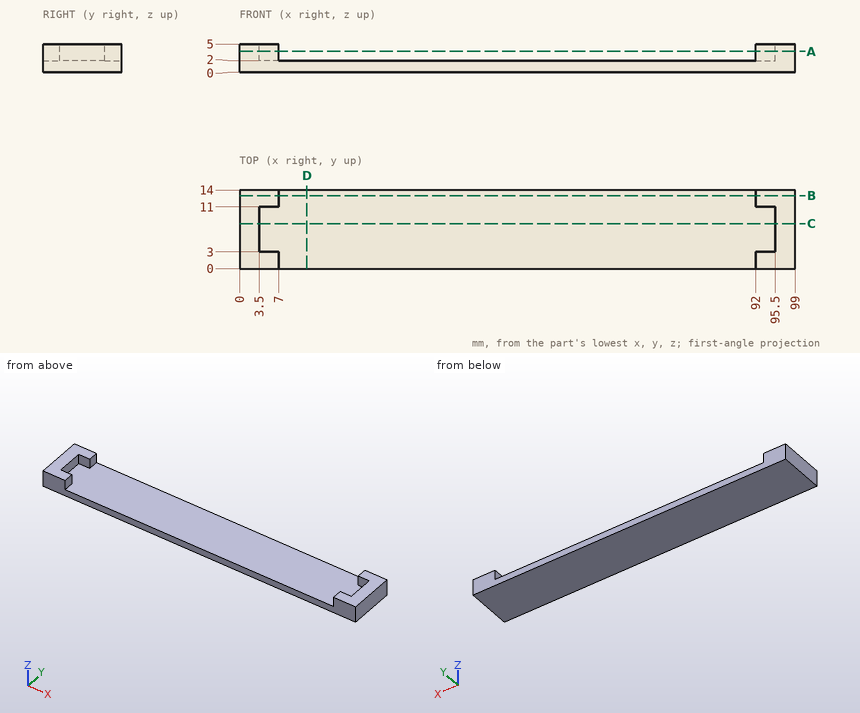
Geometry: see drawing. Coordinates: mm, zero at the bounding-box minimum. Round coordinates to 2 decimals unless told otherwise and drop trailing zeros. Loops run counter-clockwise (first coordinate to the right, second up) from the corner with the lowest first, then second, coordinate; pieces in that order, holes last. Notation, with made-up numbers: M -26,88 L -1,88 A32 cw -1,118 Z; hole C 62,12 d9. An arc over 180 degrees is marked long. Use a Markdown table: item, result. Add a question column.
1. Line query: line 1 (X direction, y = 6.5, z = 4.7); line 2 (X direction, y = 13.75, z = 4.05); line 3 (Z direction, x = 86.5, y = 8.75). Output: solid intervals per line, ascending.
2. Section query C-C on y = 8. Return the cut outline in (x, z), then the cut area to 3 significant figures.
3. Section query B-B on y = 13. Return the cut outline in (x, z), then the cut area to 3 significant figures.
4. Section query A-A on z = 3.7. Return the cut outline in (x, y), then the cut area to 3 significant figures.
5. Section query D-D on x = 12. Return the cut outline in (y, z), then the cut area to 3 significant figures.
6. Contact query for flat-ended pins moving along their axis: P1, Ø3, axis at y = 8, z = 3.5, coming from the -X side; P2, Ø5, axis at x = 87.5, y = 7.5, coming from the +Z side. Output: stop coordinate, or through.
Reported:
| question | item | result |
|---|---|---|
| 1 | line 1 | x = 0 to 3.5, 95.5 to 99 |
| 1 | line 2 | x = 0 to 7, 92 to 99 |
| 1 | line 3 | z = 0 to 2 |
| 2 | outline | M 0,0 L 99,0 L 99,5 L 95.5,5 L 95.5,2 L 3.5,2 L 3.5,5 L 0,5 Z |
| 2 | area | 219 mm² |
| 3 | outline | M 0,0 L 99,0 L 99,5 L 92,5 L 92,2 L 7,2 L 7,5 L 0,5 Z |
| 3 | area | 240 mm² |
| 4 | outline | M 0,0 L 7,0 L 7,3 L 3.5,3 L 3.5,11 L 7,11 L 7,14 L 0,14 Z; M 92,0 L 99,0 L 99,14 L 92,14 L 92,11 L 95.5,11 L 95.5,3 L 92,3 Z |
| 4 | area | 140 mm² |
| 5 | outline | M 0,0 L 14,0 L 14,2 L 0,2 Z |
| 5 | area | 28.0 mm² |
| 6 | P1 | stops at x = 0 |
| 6 | P2 | stops at z = 2 |
